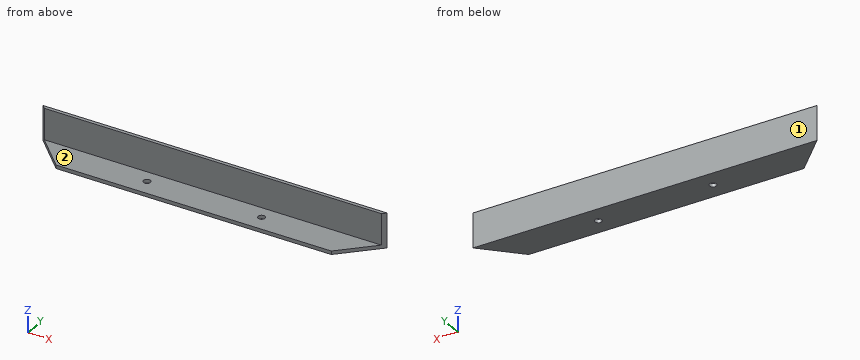
from build123d import *

# Parameters (mm, degrees)
F0_R     = 2.54
F1_DEPTH = 25.4
F2_T     = -2.54


# Not quite as in the source:
# - a feature names something its author has since deleted; it is built from what else it names


with BuildPart() as f1:
    # F0 (on Top) → F1 (new body)
    with BuildSketch(Plane.XY):
        Polygon((84.6666666667, 6.4318103081), (-169.3333333333, 6.4318103081), (-143.9333333333, -18.9681896919), (59.2666666667, -18.9681896919), align=None)
        with Locations((-84.6666666667, -6.2681896919)):
            Circle(F0_R, mode=Mode.SUBTRACT)
        with Locations((0, -6.2681896919)):
            Circle(F0_R, mode=Mode.SUBTRACT)
    extrude(amount=F1_DEPTH)

    # F2
    f2_openings = [f1.faces().sort_by_distance(p)[0] for p in [
        (71.966667, -6.26819, 12.7),
        (-156.633333, -6.26819, 12.7),
        (-42.333333, -18.96819, 12.7),
        (-42.333333, -5.794512, 25.4),
        (-87.206667, -6.26819, 12.7),
        (-2.54, -6.26819, 12.7),
    ]]
    offset(amount=F2_T, openings=f2_openings)


solid = f1.part
Read the model definition and answer for the solid it produces. Units are mm, in the model's axes. Face numbers are marked on the shaded views. A direction names the side the tool comes from. Round coordinates to 2 decimals unless told otherwise and drop trailing zeros. Write each loop counter-clockwise with the first axis right and the second up, starting at its lowest first coordinate (ties: lowest second). Pieces come first, ordered by that corner, then holes.
Q1. A tool of negligible diameter and unlimited length cuts with its end or side. For the marked faces 1 and 2, from which of +Z, -Z, +X, -X, +Y, -Y can it reach the whole face along a straight path? Write none if from no direction.
Values:
face 1: +Z, -Z, +X, -X, +Y
face 2: +Z, +X, -X, -Y
Q2. Find section C-C on z = 8. Determine the outline of the cut face in (x, y).
Values:
outline: (-169.33, 6.43) - (-166.79, 3.89) - (82.13, 3.89) - (84.67, 6.43) - close
Q3. Straight lines are drawn through the part: line 1 (Y direction, x = 0, z = 0.9); line 2 (Z direction, x = -42, y = -13.75); line 3 (Y direction, x = 74, z = 21.75). For each, find the intervals that lie inside material, in ascending order.
Values:
line 1: y = -18.97 to -8.81, -3.73 to 6.43
line 2: z = 0 to 2.54
line 3: y = 3.89 to 6.43
Q4. Find section B-B on x = -139. Determine the outline of the cut face in (y, z).
Values:
outline: (-18.97, 0) - (6.43, 0) - (6.43, 25.4) - (3.89, 25.4) - (3.89, 2.54) - (-18.97, 2.54) - close
Q5. A flat-ended cylindrical pin translates along its axis: P1, Ø5, axis at x = -56.5, z = 18, coming from the -Y side. Find the tip coordinate at first contact, or state that the pin passes through.
Values:
P1: stops at y = 3.89
Q6. Find section A-A on x = 0. Determine the outline of the cut face in (y, z), and give its area (3 significant figures).
Values:
outline: (-18.97, 0) - (-8.81, 0) - (-8.81, 2.54) - (-18.97, 2.54) - close; (-3.73, 0) - (6.43, 0) - (6.43, 25.4) - (3.89, 25.4) - (3.89, 2.54) - (-3.73, 2.54) - close
area: 110 mm2
